Part model, mm, in its own coordinate system. Coordinates: 2 decimals unless noted, no trailing zeros. Write each loop counter-clockwise with the first axis right and the second up, starting at its lowest first coordinate (ties: lowest second). Pieces come first, ordered by that corner, then holes. Notation, with made-up numbers: (-39, 87) - (18, 87) arc R5 ccw to (18, 91) - close; hole circle Ø11 at (11, -13.5). An arc over 180 degrees is marked (long way). Write each question's results on one line, items separated by ' | '.
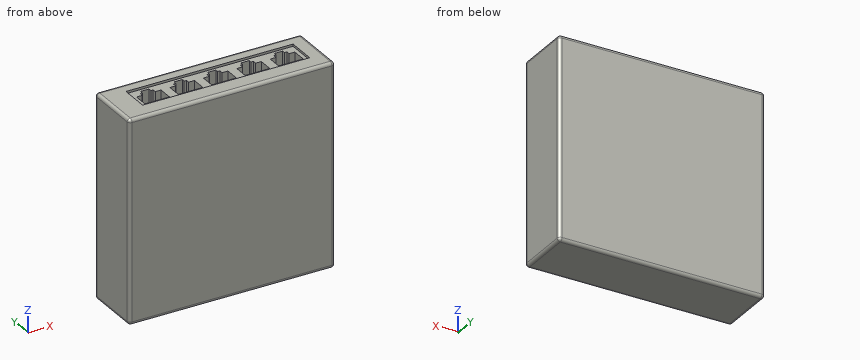
Autodesk Inventor part; units mm, degrees
ref_plane "YZ Plane" through (0, 0, 0) normal (1, 0, 0) x (0, 1, 0)
ref_plane "XZ Plane" through (0, 0, 0) normal (0, 1, 0) x (-1, 0, 0)
ref_plane "XY Plane" through (0, 0, 0) normal (0, 0, 1) x (1, 0, 0)
sketch "Sketch1" plane through (0, 0, 0) normal (0, 1, 0) x (-1, 0, 0)
  line L0 (50.2, -49.3) -> (-50.2, -49.3)
  line L1 (-50.2, -49.3) -> (-50.2, 49.3)
  line L2 (-50.2, 49.3) -> (50.2, 49.3)
  line L3 (50.2, 49.3) -> (50.2, -49.3)
  point P0 (0, 0)
  dimension "d0" = 100.4
  dimension "d1" = 98.6
  dimension "d2" = 49.3
  dimension "d3" = 50.2
extrude "Extrusion1" add sketch "Sketch1" along normal blind 28.1
sketch "Sketch2" plane through (-50.2, 0, 49.3) normal (0, 0, 1) x (1, 0, 0)
  line L0 (11.65, 22.3) -> (93.1, 22.3)
  line L1 (93.1, 22.3) -> (93.1, 8.5)
  line L2 (93.1, 8.5) -> (11.65, 8.5)
  line L3 (11.65, 8.5) -> (11.65, 22.3)
  line L4 (100.4, 0) -> (100.4, 28.1)
  line L5 (0, 0) -> (0, 28.1)
  line L6 (0, 28.1) -> (100.4, 28.1)
  line L7 (0, 0) -> (100.4, 0)
  point P0 (50.2, 0)
  point P1 (100.4, 14.05)
  dimension "d6" = 7.3
  dimension "d7" = 11.65
  dimension "d8" = 5.8
  dimension "d9" = 8.5
extrude "Extrusion2" cut sketch "Sketch2" against normal blind 1.08 contours L0 L1 L2 L3
sketch "Sketch3" plane through (-50.2, 0, 48.22) normal (0, 0, 1) x (1, 0, 0)
  line L0 (14, 17.6) -> (26, 17.6)
  line L1 (26, 17.6) -> (26, 10.65)
  line L2 (26, 10.65) -> (14, 10.65)
  line L3 (14, 10.65) -> (14, 17.6)
  line L4 (16.825, 19.4) -> (23.175, 19.4)
  line L5 (23.175, 19.4) -> (23.175, 17.6)
  line L6 (23.175, 17.6) -> (16.825, 17.6)
  line L7 (16.825, 17.6) -> (16.825, 19.4)
  line L8 (17.95, 20.92) -> (22.05, 20.92)
  line L9 (22.05, 20.92) -> (22.05, 19.4)
  line L10 (22.05, 19.4) -> (17.95, 19.4)
  line L11 (17.95, 19.4) -> (17.95, 20.92)
  line L12 (93.1, 8.5) -> (11.65, 8.5)
  line L13 (11.65, 8.5) -> (11.65, 22.3)
  point P0 (50.2, 0)
  point P1 (17.95, 19.4)
  dimension "d12" = 12
  dimension "d13" = 6.35
  dimension "d14" = 4.1
  dimension "d15" = 2.825
  dimension "d16" = 2.825
  dimension "d17" = 1.125
  dimension "d18" = 1.125
  dimension "d19" = 6.95
  dimension "d20" = 1.8
  dimension "d21" = 1.52
  dimension "d22" = 2.15
  dimension "d23" = 2.35
extrude "Extrusion3" cut sketch "Sketch3" against normal blind 11.78
pattern_linear "Rectangular Pattern1" count 5 spacing 16.3 along (1, 0, 0) of "Extrusion3"
fillet "Fillet1" radius 1.5 12 edges at (0, 28.1, -49.3) (-50.2, 28.1, 0) (0, 28.1, 49.3) (50.2, 28.1, 0) (50.2, 14.05, 49.3) (-50.2, 14.05, 49.3) (-50.2, 14.05, -49.3) (-50.2, 0, 0) (0, 0, -49.3) (50.2, 14.05, -49.3) (50.2, 0, 0) (0, 0, 49.3)
properties part number "5-port-switch"
(1) Wall check: line 1 (Z direction, x = -3, y = 14.5); line 2 (Z direction, x = -7, y = 16.5). Give the ranges that are in metal, low to high. Write a range as from..to.
Return value:
line 1: z = -49.3..36.44 | line 2: z = -49.3..48.22
(2) Saw through at B-B on x = -13.5. Write the cut outline in (y, z).
Return value:
outline: (0, -47.8) arc R1.5 ccw to (1.5, -49.3) - (26.6, -49.3) arc R1.5 ccw to (28.1, -47.8) - (28.1, 47.8) arc R1.5 ccw to (26.6, 49.3) - (22.3, 49.3) - (22.3, 48.22) - (20.92, 48.22) - (20.92, 36.44) - (10.65, 36.44) - (10.65, 48.22) - (8.5, 48.22) - (8.5, 49.3) - (1.5, 49.3) arc R1.5 ccw to (0, 47.8) - close
(3) Flat gauge pins, fed straight in: P1, Ø0.5, axis at x = 14, z = 48.5, coming from the -Y side; P2, Ø3, axis at x = -28, y = 16, coming from the +Z side. Where does each tip first touch, or does it go through?
Return value:
P1: stops at y = 0.07 | P2: stops at z = 36.44
